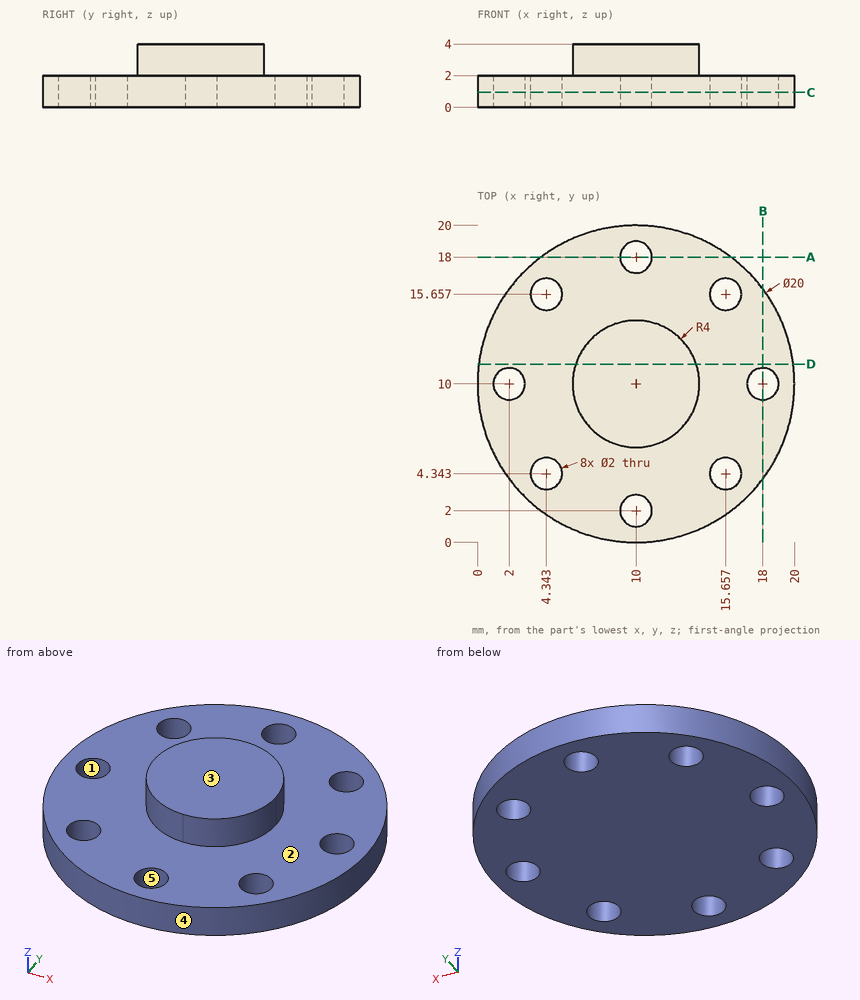
Study the drawing (mm; zero at the part's minimum x, y, z) and answer. A direction names the side the tool comes from. Coordinates: 2 decimals unless noted, no trailing zeros. Loops run counter-clockwise (first coordinate to the right, second up) from the corner with the lowest first, then second, coordinate; pieces in that order, holes last. Notation, with made-up numbers: M 30.5,88 L 35.5,88 A9 ccw 35.5,100 Z; hole C 72,80.5 d10. An arc over 180 degrees is marked long. Answer in a Markdown table with one row per item. Add a question column.
1. Consider L1, parallel to Y at x = 10, z = 1.2; L2, parallel to Y at x = 15.75, z = 1.2; L3, parallel to Z at x = 7, y = 16.25. Determine where each line is inside the solid, lowest interval first.
2. Flat-ended cylindrical pins translate along their axes: P1, Ø1.5, axis at y = 3.5, z = 2.5, coming from the +X side; P2, Ø2.5, axis at x = 4.34, y = 15.66, coming from the +Z side. Find the tip coordinate at first contact, or state that the pin passes through.
3. The mould has two halves that part along Y. Classify the marked faces 3, 4 and 5: pulls with the +Y half, pulls with the -Y half, needs draft (parallel to the pull), parting line crosses it, or undercut.
4. A tool of negligible diameter and unlimited length cuts with its end or side. For the marked faces 1 and 2, from which of +Z, -Z, +X, -X, +Y, -Y can it reach the whole face along a straight path? Write none if from no direction.
5. Find section D-D, the plane y = 11.25. Write down the section's boundary in (x, z), then the cut area to 3 significant figures.
6. Find section C-C, the plane z = 0.95. State how many separate pieces and enclosed holes the cut face has, then the cut area to 3 significant figures.
7. Find section A-A, the plane y = 18. Write down the section's boundary in (x, z).
Reported:
| question | item | result |
|---|---|---|
| 1 | L1 | y = 0 to 1, 3 to 17, 19 to 20 |
| 1 | L2 | y = 1.82 to 3.35, 5.34 to 14.66, 16.65 to 18.18 |
| 1 | L3 | z = 0 to 2 |
| 2 | P1 | stops at x = 18.04 |
| 2 | P2 | stops at z = 2 |
| 3 | face 3 | needs draft |
| 3 | face 4 | parting line crosses it |
| 3 | face 5 | undercut |
| 4 | face 1 | +Z, -Z |
| 4 | face 2 | +Z |
| 5 | outline | M 0.08,0 L 19.92,0 L 19.92,2 L 13.8,2 L 13.8,4 L 6.2,4 L 6.2,2 L 0.08,2 Z |
| 5 | area | 54.9 mm^2 |
| 6 | separate pieces | 1 |
| 6 | enclosed holes | 8 |
| 6 | area | 289 mm^2 |
| 7 | outline | M 4,0 L 9,0 L 9,2 L 4,2 Z; M 11,0 L 16,0 L 16,2 L 11,2 Z |
